For this review, take the finished solid that the model builds, in its own axes (mm). A direction names the side the tool comes from. Coordinates: 2 decimals unless noted, no trailing zeros. Loops run counter-clockwise (first coordinate to the right, second up) from the corner with the lowest first, then second, coordinate; pieces in that order, holes last. Notation, with made-up numbers: (-15.5, -36) - (30.5, -36) arc R25 cw to (30.5, -11) - close; hole circle Ø3 at (14, -14.5). An arc over 180 degrees is marked (long way). One line per item, written item: value. Start each with the question number.
1. Insertion check: pin 1 (8 mm diameter, centred on y = -27, z = 18, fed in from +X); pin 2 (6 mm diameter, centred on x = 0, y = -16.5, fed in from +Z); pin 3 (1 mm diameter, centred on y = -16.5, z = 21.5, fed in from -X). Each pin has a flat end and moves straight along its axis. Give the tip position at first contact, or say it passes through.
2. Take a section at A-A, the plane y = -12. State the section outline as (x, z) points, and give its area (3 significant figures).
3. Take a section at C-C, the plane x = -7. State the section outline as (y, z) points.
4. The part is to be moulded in two halves that separate along Y. For faces 1 (the face through (0, -30, 1)), 2 (the face through (-27.766, -14.79, 17.422)), 3 (the face through (31, -2.25, 32)), say which applies: released by +Y, released by -Y, zero draft, split by the parting line, or undercut.
5. To check wall thickness, follow line 1 (Z direction, x = -9.5, y = -10); line 2 (X direction, y = -7.75, z = 20.5); line 3 (X direction, y = -13.25, z = 24). State the ranges of each line that lie inside material, in increasing order. Write a range as from..to.
6. For faces 4 (the face through (30.153, -15.178, 27.122)), 5 (the face through (0, -15, 2)), 6 (the face through (31.61, -15.18, 37.52)), 7 (the face through (-30.153, -14.822, 27.122)), list the 3-axis set-ups (+Z, -Z, +X, -X, +Y, -Y) from which the entire face can be reached by the end or side of a thin tool; tool diameter is ignored.
7. Take a section at B-B, the plane z = 16. State the section outline as (x, y) points, and give its area (3 significant figures).
```python
from build123d import *

# Parameters (mm, degrees)
F1_DEPTH = 30
F2_W     = 25.5
F2_H     = 10.5
F3_DEPTH = 5
F4_W     = 25.5
F4_H     = 10.5
F5_DEPTH = 5


with BuildPart() as f1:
    # F0 (on Front) → F1 (new body)
    with BuildSketch(Plane.XZ):
        Polygon((0.0016284716, 2), (-0.0016284716, 2), (-25.5983715284, 2), (-31.2740161038, 42.3843095671), (-33.2866138074, 42.3340932619), (-27.336945004, 0), (0, 0), (27.336945004, 0), (33.2866138074, 42.3340932619), (31.2740161038, 42.3843095671), (25.5983715284, 2), align=None)
    extrude(amount=F1_DEPTH)

    # F2 (on face) → F3 (cut)
    with BuildSketch(Plane(origin=(26.8074515602, 0, -3.7675416185), x_dir=(0, 1, 0), z_dir=(0.9902680687, 0, -0.139173101))):
        with Locations((-15, 36.3047020404)):
            Rectangle(F2_W, F2_H)
    extrude(amount=-F3_DEPTH, mode=Mode.SUBTRACT)

    # F4 (on face) → F5 (cut)
    with BuildSketch(Plane(origin=(-26.8074515602, 0, -3.7675416185), x_dir=(0, -1, 0), z_dir=(-0.9902680687, 0, -0.139173101))):
        with Locations((15, 36.3047020404)):
            Rectangle(F4_W, F4_H)
    extrude(amount=-F5_DEPTH, mode=Mode.SUBTRACT)


solid = f1.part
```
Solutions:
1. pin 1: x = 30.43
1. pin 2: z = 2
1. pin 3: x = -30.43
2. outline: (-33.29, 42.33) - (-32.59, 37.38) - (-30.61, 37.66) - (-31.27, 42.38) - close; (-31.13, 26.98) - (-27.34, 0) - (27.34, 0) - (31.13, 26.98) - (29.15, 27.26) - (25.6, 2) - (-25.6, 2) - (-29.15, 27.26) - close; (30.61, 37.66) - (32.59, 37.38) - (33.29, 42.33) - (31.27, 42.38) - close
2. area: 231 mm2
3. outline: (-30, 0) - (0, 0) - (0, 2) - (-30, 2) - close
4. face 1: released by -Y
4. face 2: zero draft
4. face 3: undercut
5. line 1: 0..2
5. line 2: -30.22..-28.2, 28.2..30.22
5. line 3: -30.71..-28.69, 28.69..30.71
6. face 4: +X
6. face 5: +Z, +Y, -Y
6. face 6: none
6. face 7: -X
7. outline: (-29.59, -30) - (-27.57, -30) - (-27.57, 0) - (-29.59, 0) - close; (27.57, -30) - (29.59, -30) - (29.59, 0) - (27.57, 0) - close
7. area: 121 mm2
